from build123d import *

# Parameters (mm, degrees)
BOSS_EXTRUDE1_DEPTH = 1.6
SKETCH3_R           = 1
BOSS_EXTRUDE2_DEPTH = 9


with BuildPart() as part:
    # Sketch1 → Boss-Extrude1 (new body)
    with BuildSketch(Plane.XY):
        with BuildLine():
            Line((-41.383181355, 43.426165336), (-41.383181355, 7.477968892))
            Line((-41.383181355, 7.477968892), (-45.94349159, 7.477968892))
            Line((-45.94349159, 7.477968892), (-45.94349159, -3.396104602))
            Line((-45.94349159, -3.396104602), (-66.113144039, -3.396104602))
            Line((-66.113144039, -3.396104602), (-66.113144039, 40.440533192))
            ThreePointArc((-66.113144039, 40.440533192), (-65.656687939, 42.166215415), (-64.406709132, 43.4405326))
            Line((-64.406709132, 43.4405326), (-41.383181355, 43.426165336))
        make_face()
    extrude(amount=BOSS_EXTRUDE1_DEPTH)

    # Sketch3 → Boss-Extrude2 (add)
    with BuildSketch(Plane(origin=(0, 0, 0), x_dir=(-1, 0, 0), z_dir=(0, 0, -1))):
        with Locations((50.189000543, 0)):
            Circle(SKETCH3_R)
        with Locations((60.928928446, 0)):
            Circle(SKETCH3_R)
        with Locations((64.113441952, 40.81521395)):
            Circle(SKETCH3_R)
    extrude(amount=BOSS_EXTRUDE2_DEPTH)


solid = part.part
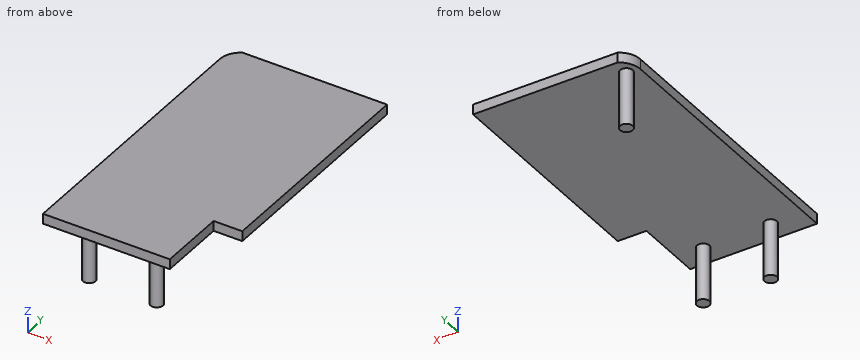
Geometry check sheet. Reference: the model listing, model coordinates, mm. Give positions to 0.01 mm unless a question says otherwise; leave off trailing zeros. Loops run counter-clockwise (first coordinate to the right, second up) from the corner with the lowest first, then second, coordinate; pieces in that order, holes last. Notation, with made-up numbers: (-21.5, 55.5) -> (23.5, 55.5) arc R29 ccw to (23.5, 76.5) -> close; hole circle Ø8 at (33, 39.5). An arc over 180 degrees is marked (long way). Answer in a Markdown table with one row per item. Add a question column.
1) Cross-section at C-C on z = -2. Record the boundary of the cut face in (x, y), and give its area (3 significant figures).
2) Cross-section at D-D on y = 17. Record the boundary of the cut face in (x, z), and give its area (3 significant figures).
3) Material ranges on probe 1 along Z at (x, y) = (-60.5, 18); probe 2 along Y at (x, z) = (-53.75, 0.75); probe 3 along Y at (x, z) = (-64.25, -4.75), recorded low to high. Write a range as from..to.
4) Cross-section at A-A on y = 0. Record the boundary of the cut face in (x, z), and give its area (3 significant figures).
5) Gauge pin test, flat ends, axial feed: P1, Ø1, axis at x = -49, z = -1, coming from the -Y side; P2, Ø3, axis at x = -59.5, y = 36.5, coming from the -Z side; P3, Ø1.5, axis at x = -60.5, z = -6.5, coming from the -Y side; P4, Ø1.5, axis at y = 34.5, z = -1.5, coming from the -X side. Record the tip position at first contact, or that the pin passes through.
6) Cross-section at B-B on x = -61. Record the boundary of the cut face in (y, z), and give its area (3 significant figures).
Outcome:
| question | item | result |
|---|---|---|
| 1 | outline | circle Ø2 at (-64.11, 40.82); circle Ø2 at (-60.93, 0); circle Ø2 at (-50.19, 0) |
| 1 | area | 9.42 mm^2 |
| 2 | outline | (-66.11, 0) -> (-41.38, 0) -> (-41.38, 1.6) -> (-66.11, 1.6) -> close |
| 2 | area | 39.6 mm^2 |
| 3 | probe 1 | z = 0..1.6 |
| 3 | probe 2 | y = -3.4..43.43 |
| 3 | probe 3 | y = 39.82..41.81 |
| 4 | outline | (-66.11, 0) -> (-61.93, 0) -> (-61.93, -9) -> (-59.93, -9) -> (-59.93, 0) -> (-51.19, 0) -> (-51.19, -9) -> (-49.19, -9) -> (-49.19, 0) -> (-45.94, 0) -> (-45.94, 1.6) -> (-66.11, 1.6) -> close |
| 4 | area | 68.3 mm^2 |
| 5 | P1 | stops at y = -0.72 |
| 5 | P2 | stops at z = 0 |
| 5 | P3 | stops at y = -1 |
| 5 | P4 | passes through |
| 6 | outline | (-3.4, 0) -> (-1, 0) -> (-1, -9) -> (1, -9) -> (1, 0) -> (43.44, 0) -> (43.44, 1.6) -> (-3.4, 1.6) -> close |
| 6 | area | 92.9 mm^2 |
